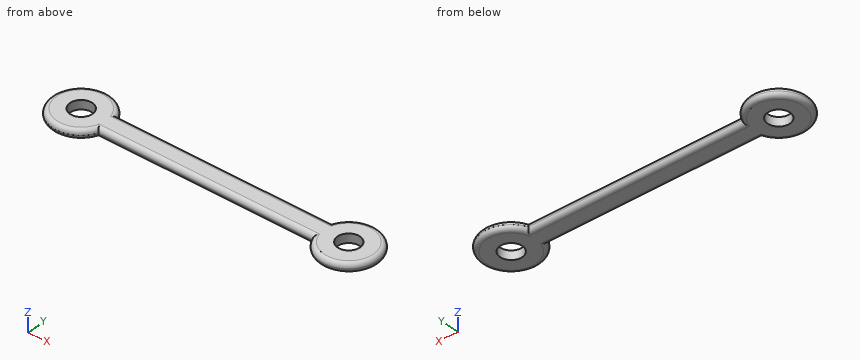
```python
from build123d import *

# Parameters (mm, degrees)
SKETCH1_R           = 6.35
BOSS_EXTRUDE1_DEPTH = 5.08
FILLET1_R           = 2.54
FILLET2_R           = 2.54


with BuildPart() as part:
    # Sketch1 → Boss-Extrude1 (new body)
    with BuildSketch(Plane.XY):
        with BuildLine():
            Line((15.24, -6.35), (137.16, -6.35))
            ThreePointArc((137.16, -6.35), (168.91, 0), (137.16, 6.35))
            Line((137.16, 6.35), (15.24, 6.35))
            ThreePointArc((15.24, 6.35), (-16.51, 0), (15.24, -6.35))
        make_face()
        Circle(SKETCH1_R, mode=Mode.SUBTRACT)
        with Locations((152.4, 0)):
            Circle(SKETCH1_R, mode=Mode.SUBTRACT)
    extrude(amount=BOSS_EXTRUDE1_DEPTH)

    # Fillet1
    fillet1_edges = [part.edges().sort_by_distance(p)[0] for p in [
        (-16.51, 0, 5.08),
        (76.2, -6.35, 5.08),
        (168.91, 0, 5.08),
        (76.2, 6.35, 5.08),
    ]]
    fillet(fillet1_edges, radius=FILLET1_R)

    # Fillet2
    fillet2_edges = [part.edges().sort_by_distance(p)[0] for p in [
        (76.2, -6.35, 0),
        (-16.51, 0, 0),
        (76.2, 6.35, 0),
        (168.91, 0, 0),
    ]]
    fillet(fillet2_edges, radius=FILLET2_R - 0.0001)  # a hair under: the kernel refuses the full size


solid = part.part
```
Model file for the job. Use its own axes, mm. Coordinates: 2 decimals unless noted, no trailing zeros. Write each loop counter-clockwise with the first axis right and the second up, starting at its lowest first coordinate (ties: lowest second). Pieces come first, ordered by that corner, then holes. Notation, with made-up numbers: (18, -29.5) - (69, -29.5) arc R20 ccw to (69, -18.5) - close; hole circle Ø1 at (82, -30.75). An arc over 180 degrees is marked (long way). One line per question, with ' | ' between items. Start each with the question number.
Q1. Cut at D-D, the plane z = 1.4. List the corners of the cut face in (x, y).
Q2. Cut at B-B, the plane y = 0. Give the number of separate pieces and of enclosed holes in the cut face, then the cut area to 3 significant figures.
Q3. Pin check, flat tips, straight feed: pin 1 (3 mm diameter, centred on y = 13, z = 2, fed in from +X); pin 2 (1 mm diameter, centred on x = 75.5, z = 3, fed in from -Y); pin 3 (5 mm diameter, centred on x = 109.5, y = 8, fed in from -Z). Stop position of each tip, or through.
Q4. Drill centre lines: line 1 (X direction, y = 2, z = 3.55); line 2 (Y direction, x = 0, z = 3.65); line 3 (X direction, y = -5, z = 4.7). Where is each one in solid material? Low to high. Write a range as [from, to].
Answer below:
1) outline: (15.06, -6.08) - (137.34, -6.08) arc R16.24 ccw (long way) to (137.34, 6.08) - (15.06, 6.08) arc R16.24 ccw (long way) to start; hole circle Ø12.7 at (0, 0); hole circle Ø12.7 at (152.4, 0)
2) separate pieces: 3 | enclosed holes: 0 | area: 807 mm^2
3) pin 1: x = 164.2 | pin 2: y = -6.35 | pin 3: z = 0.64
4) line 1: [-16.18, -6.03], [6.03, 146.37], [158.43, 168.58] | line 2: [-16.25, -6.35], [6.35, 16.25] | line 3: [-14.47, -3.91], [3.91, 148.49], [156.31, 166.87]
